Autodesk Inventor part; units mm, degrees
ref_plane "YZ Plane" through (0, 0, 0) normal (1, 0, 0) x (0, 1, 0)
ref_plane "XZ Plane" through (0, 0, 0) normal (0, 1, 0) x (-1, 0, 0)
ref_plane "XY Plane" through (0, 0, 0) normal (0, 0, 1) x (1, 0, 0)
sketch "Sketch1" plane through (0, 0, 0) normal (0, 1, 0) x (-1, 0, 0)
  line L0 (0, 0) -> (-69, 0)
  line L1 (-69, 0) -> (-69, 69)
  line L2 (-69, 69) -> (0, 69)
  line L3 (0, 69) -> (0, 0)
  circle A0 centre (-34.5, 30) radius 17
  dimension "d0" = 69
  dimension "d1" = 69
  dimension "d2" = 34
  dimension "d5" = 30
extrude "Extrusion1" add sketch "Sketch1" along normal blind 3
properties part number "field-mover-motor-case"
Geometry: final body of the model. Coordinates: model frame, mm. Round coordinates to 2 decimals unless told otherwise and drop trailing zeros. Loops run counter-clockwise (first coordinate to the right, second up) from the corner with the lowest first, then second, coordinate; pieces in that order, holes last. Notation, with made-up numbers: M 0,7 L 35,7 A19 ccw 35,35 Z; hole C -10,17.5 d4. An arc over 180 degrees is marked long. One line per question, with ' | ' between items.
(1) Cut plane A-A on z = 30. Return the cut outline in (x, y), plus the area to 3 significant figures.
Check result:
outline: M 0,0 L 17.5,0 L 17.5,3 L 0,3 Z; M 51.5,0 L 69,0 L 69,3 L 51.5,3 Z | area: 105 mm2
(2) Cut plane C-C on x = 34.5. Return the cut outline in (y, z), plus the area to 3 significant figures.
Check result:
outline: M 0,0 L 3,0 L 3,13 L 0,13 Z; M 0,47 L 3,47 L 3,69 L 0,69 Z | area: 105 mm2
(3) Material intervals for line 1 along Z through (x, y) = (34.5, 1.9); line 2 along X through (y, z) = (1, 21); line 3 along Z through (x, y) = (20.5, 2.05), sorted ascending. Write a range as from..to.
Check result:
line 1: z = 0..13, 47..69 | line 2: x = 0..20.08, 48.92..69 | line 3: z = 0..20.36, 39.64..69
(4) Pull-direction query (Z, two-part tool) for faces 1 (the cylindrical face through (38.185, 1.479, 46.596)), 2 (the flat face through (34, 1, 0)), 3 (the flat face through (35, 1, 69)), 4 (the flat face through (35, 0, 50)); classes: +Z half, -Z half, draft (parallel to the pull), parting line (faces both ways), or undercut.
Check result:
face 1: undercut | face 2: -Z half | face 3: +Z half | face 4: draft
(5) Cut plane B-B on y = 1.05. Return the cut outline in (x, z), plus the area to 3 significant figures.
Check result:
outline: M 0,0 L 69,0 L 69,69 L 0,69 Z; hole C 34.5,30 d34 | area: 3,850 mm2
(6) Contact query for a flat-ended pin moving along its axis: P1, Ø12, axis at x = 45.5, z = 9, coming from the -Y side. Output: stop coordinate, or through.
Check result:
P1: stops at y = 0
